Read the model definition and answer for the solid it produces. Units are mm, in the model's axes. Coordinates: 2 decimals unless noted, no trailing zeros. Loops run counter-clockwise (first coordinate to the right, second up) from the corner with the lowest first, then second, coordinate; pieces in that order, holes last. Notation, with made-up numbers: (-8.75, -30.5) -> (-1.75, -30.5) arc R27 ccw to (-1.75, -7.5) -> close; hole circle Ø10 at (53.25, 88.25). An arc over 180 degrees is marked (long way). Answer as CSV lines item,"result".
```python
from build123d import *

# Parameters (mm, degrees)
BOSS_EXTRUDE1_DEPTH = 3.175
SKETCH2_W           = 2.794
SKETCH2_H           = 38.1
CUT_EXTRUDE1_DEPTH  = 3.175
FILLET1_R           = 3.175
SKETCH3_W           = 2.794
SKETCH3_H           = 38.1
CUT_EXTRUDE2_DEPTH  = 9.525
SKETCH4_W           = 2.794
SKETCH4_H           = 38.1
CUT_EXTRUDE3_DEPTH  = 3.175


with BuildPart() as part:
    # Sketch1 → Boss-Extrude1 (new body)
    with BuildSketch(Plane(origin=(0, 0, 0), x_dir=(1, 0, 0), z_dir=(0, 1, 0))):
        Polygon((50.8, 30.1625), (101.6, 30.1625), (101.6, -30.1625), (-101.6, -30.1625), (-101.6, 30.1625), (-50.8, 30.1625), (-50.8, 71.4375), (50.8, 71.4375), align=None)
    extrude(amount=BOSS_EXTRUDE1_DEPTH)

    # Sketch2 → Cut-Extrude1 (cut)
    with BuildSketch(Plane(origin=(0, 3.175, 0), x_dir=(1, 0, 0), z_dir=(0, 1, 0))):
        with Locations((4.572, 33.3375)):
            Rectangle(SKETCH2_W, SKETCH2_H)
    extrude(amount=-CUT_EXTRUDE1_DEPTH, mode=Mode.SUBTRACT)

    # Fillet1
    fillet1_edges = [part.edges().sort_by_distance(p)[0] for p in [
        (101.6, 1.5875, 30.1625),
        (-101.6, 1.5875, 30.1625),
        (-101.6, 1.5875, -30.1625),
        (-50.8, 1.5875, -30.1625),
        (-50.8, 1.5875, -71.4375),
        (50.8, 1.5875, -71.4375),
        (50.8, 1.5875, -30.1625),
        (101.6, 1.5875, -30.1625),
    ]]
    fillet(fillet1_edges, radius=FILLET1_R)

    # Sketch3 → Cut-Extrude2 (cut)
    with BuildSketch(Plane(origin=(0, 3.175, 0), x_dir=(1, 0, 0), z_dir=(0, 1, 0))):
        with Locations((-36.3855, 33.3375)):
            Rectangle(SKETCH3_W, SKETCH3_H)
    extrude(amount=-CUT_EXTRUDE2_DEPTH, mode=Mode.SUBTRACT)

    # Sketch4 → Cut-Extrude3 (cut)
    with BuildSketch(Plane(origin=(0, 3.175, 0), x_dir=(1, 0, 0), z_dir=(0, 1, 0))):
        with Locations((42.672, 33.3375)):
            Rectangle(SKETCH4_W, SKETCH4_H)
    extrude(amount=-CUT_EXTRUDE3_DEPTH, mode=Mode.SUBTRACT)


solid = part.part
```
Q1. A cutting plane is placed at C-C, the plane z = -64. Write down the section's boundary in (x, y) (3 decimals), and give its area (3 significant figures).
Results:
outline,"(-50.8, 0) -> (50.8, 0) -> (50.8, 3.175) -> (-50.8, 3.175) -> close"
area,"323 mm²"
Q2. Given pin 1 Ø1.6 at (y, z) = (1, -50) entering from -X; pin 2 Ø1 at (y, z) = (2, -36) entering from +X; pin 3 Ø1.6 at (y, z) = (1.5, -30) entering from -X, each flat-ended and moving along its own axis, determine where each tip first touches the part or whether it passes through.
Results:
pin 1,"stops at x = -50.8"
pin 2,"stops at x = 50.8"
pin 3,"stops at x = -100.7"
Q3. A cutting plane is placed at D-D, the plane x = 67. Write down the section's boundary in (y, z) (1 decimal).
Results:
outline,"(0, -30.2) -> (3.2, -30.2) -> (3.2, 30.2) -> (0, 30.2) -> close"
Q4. A cutting plane is placed at A-A, the plane z = -49. Write down the section's boundary in (x, y) (1 decimal), and give its area (3 significant figures).
Results:
outline,"(-50.8, 0) -> (-37.8, 0) -> (-37.8, 3.2) -> (-50.8, 3.2) -> close; (-35, 0) -> (3.2, 0) -> (3.2, 3.2) -> (-35, 3.2) -> close; (6, 0) -> (41.3, 0) -> (41.3, 3.2) -> (6, 3.2) -> close; (44.1, 0) -> (50.8, 0) -> (50.8, 3.2) -> (44.1, 3.2) -> close"
area,"296 mm²"
Q5. A cutting plane is placed at B-B, the plane y = 2.2. Give the number of separate pieces and of enclosed holes in the cut face, and give its area (3 significant figures).
Results:
separate pieces,"1"
enclosed holes,"3"
area,"16,100 mm²"
Q6. Find the intervals of material crossed by probe 1 along X at (y, z) = (2.75, -19) (1 decimal); probe 2 along X at (y, z) = (0.2, -39) (1 decimal); probe 3 along Z at (x, y) = (5, 0.4), in increasing order. Write a range as [from, to].
Results:
probe 1,"x = [-101.6, -37.8], [-35, 3.2], [6, 41.3], [44.1, 101.6]"
probe 2,"x = [-50.8, -37.8], [-35, 3.2], [6, 41.3], [44.1, 50.8]"
probe 3,"z = [-71.44, -52.39], [-14.29, 30.16]"
